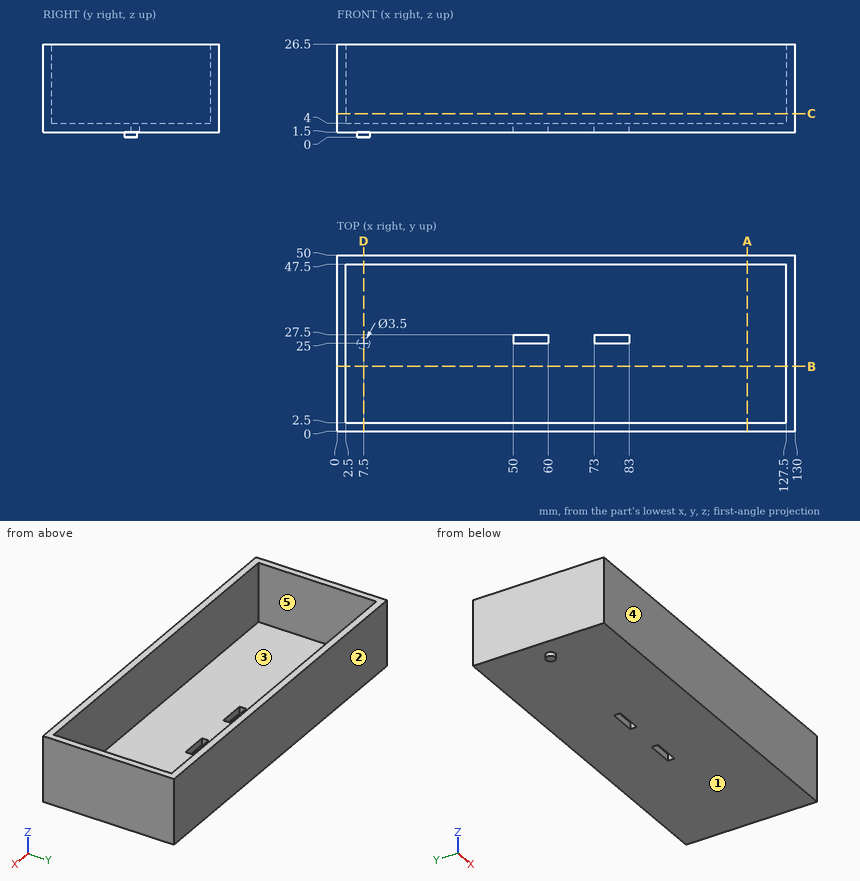
Here's the drawing with two shaded views (mm, measured from the low corner). I have some questions. A direction names the side the tool comes from. Coordinates: 2 decimals unless noted, no trailing zeros. Write each loop counter-clockwise with the first axis right and the second up, starting at its lowest first coordinate (ties: lowest second). Pieces come first, ordered by that corner, then holes. Notation, with made-up numbers: (-20, 31.25) -> (28, 31.25) arc R26 ccw to (28, 64.25) -> close; hole circle Ø9 at (36, 0.25). An arc over 180 degrees is marked (long way). Answer as CSV lines item,"result".
1) If we section it at A-A on x = 116.5: Please give me the cut outline in (y, z), then the cut area to 4 significant figures.
Check result:
outline,"(0, 1.5) -> (50, 1.5) -> (50, 26.5) -> (47.5, 26.5) -> (47.5, 4) -> (2.5, 4) -> (2.5, 26.5) -> (0, 26.5) -> close"
area,"237.5 mm²"
2) If we section it at B-B on y = 18.5: Please give me the cut outline in (x, z).
Check result:
outline,"(0, 1.5) -> (130, 1.5) -> (130, 26.5) -> (127.5, 26.5) -> (127.5, 4) -> (2.5, 4) -> (2.5, 26.5) -> (0, 26.5) -> close"
3) If we mould it in two halves opening along Y, with no side actions, what happens to the marked faces 1, 2 and 3? For each: +Y half, -Y half, draft (parallel to the pull), parting line (faces both ways), or undercut.
Check result:
face 1,"draft"
face 2,"+Y half"
face 3,"undercut"
4) Will these pins go through, and if not, where does the flat tip stop? P1, Ø10, axis at x = 113.5, y = 30, coming from the +Z side; P2, Ø2, axis at x = 112, y = 13.5, coming from the -Z side; P3, Ø11, axis at y = 14.5, z = 10.5, coming from the -X side.
Check result:
P1,"z = 4"
P2,"z = 1.5"
P3,"x = 0"
5) If I drill on line 1 (Y direction, x = 7.5, z = 14.75); line 2 (X direction, y = 24, z = 7.25); line 3 (Z direction, x = 110, y = 2), over which ranges is the centre line in solid material (lowest first)? Write a range as from..to.
Check result:
line 1,"0..2.5, 47.5..50"
line 2,"0..2.5, 127.5..130"
line 3,"1.5..26.5"
6) On a 3-axis mill with a long thin cutter (end or side, diameter ignored), from which of +Z, -Z, +X, -X, +Y, -Y can I reach the whole of each face in a straight line? I mean the marked faces 4 and 5. Say none if no direction works.
Check result:
face 4,"+Z, -Z, +X, -X, -Y"
face 5,"+Z"
7) If we section it at C-C on z = 6.75: Please give me the cut outline in (x, y), then the cut area to 3 significant figures.
Check result:
outline,"(0, 0) -> (130, 0) -> (130, 50) -> (0, 50) -> close; hole (2.5, 2.5) -> (127.5, 2.5) -> (127.5, 47.5) -> (2.5, 47.5) -> close"
area,"875 mm²"
8) If we section it at D-D on x = 7.5: Please give me the cut outline in (y, z), then the cut area to 3 significant figures.
Check result:
outline,"(0, 1.5) -> (23.25, 1.5) -> (23.25, 0) -> (26.75, 0) -> (26.75, 1.5) -> (50, 1.5) -> (50, 26.5) -> (47.5, 26.5) -> (47.5, 4) -> (2.5, 4) -> (2.5, 26.5) -> (0, 26.5) -> close"
area,"243 mm²"
